Input: dimensioned drawing with shaded views. Units: mm. Origin: part minimum x, y, z. A direction names the side the tool comes from. Coordinates: 2 decimals unless noted, no trailing zeros. Write each loop counter-clockwise with the first axis right and the second up, starting at its lowest first coordinate (ties: lowest second). Pieces come first, ordered by that corner, then holes. Notation, with made-up numbers: M 60.25,10.25 L 88.25,10.25 A31 ccw 88.25,38.25 Z; hole C -33,63 d2. An arc over 180 degrees is marked long. Write each question's results on one line, items separated by ' | '. Start each with the question number.
1. First-contact query: pin 1 (4 mm diameter, centred on x = 4, y = 20.5, fed in from +Z); pin 2 (1 mm diameter, centred on x = 2, z = 33.5, fed in from +Y); pin 3 (5 mm diameter, centred on x = 4.5, y = 25, fed in from +Z). Flat tips, straight axial feed; report the tip coordinate or a pass-through.
2. Pull-direction query (Y, two-part tool) for the marked faces 1, 2 and 3; classes: +Y half, -Y half, draft (parallel to the pull), parting line (faces both ways), or undercut.
3. Section query D-D, the plane z = 30. Output: boundary loops of the cut face in (x, y), and give its area (3 significant figures).
4. Section query C-C, the plane x = 5.25. Output: boundary loops of the cut face in (y, z).
5. Section query A-A, the plane y = 20. Output: boundary loops of the cut face in (x, z).
6. Ray query, probe 1 along Y at (x, z) = (2.5, 20); probe 2 along Y at (x, z) = (6.5, 20); probe 3 along X at (y, z) = (26, 2). Return the intervals inside material, ascending.
7. Set-up query: the marked faces 4 and 5. Return all of +Z, -Z, +X, -X, +Y, -Y with unobstructed straight access to the full face (end or side cutting, diameter ignored); none if empty.
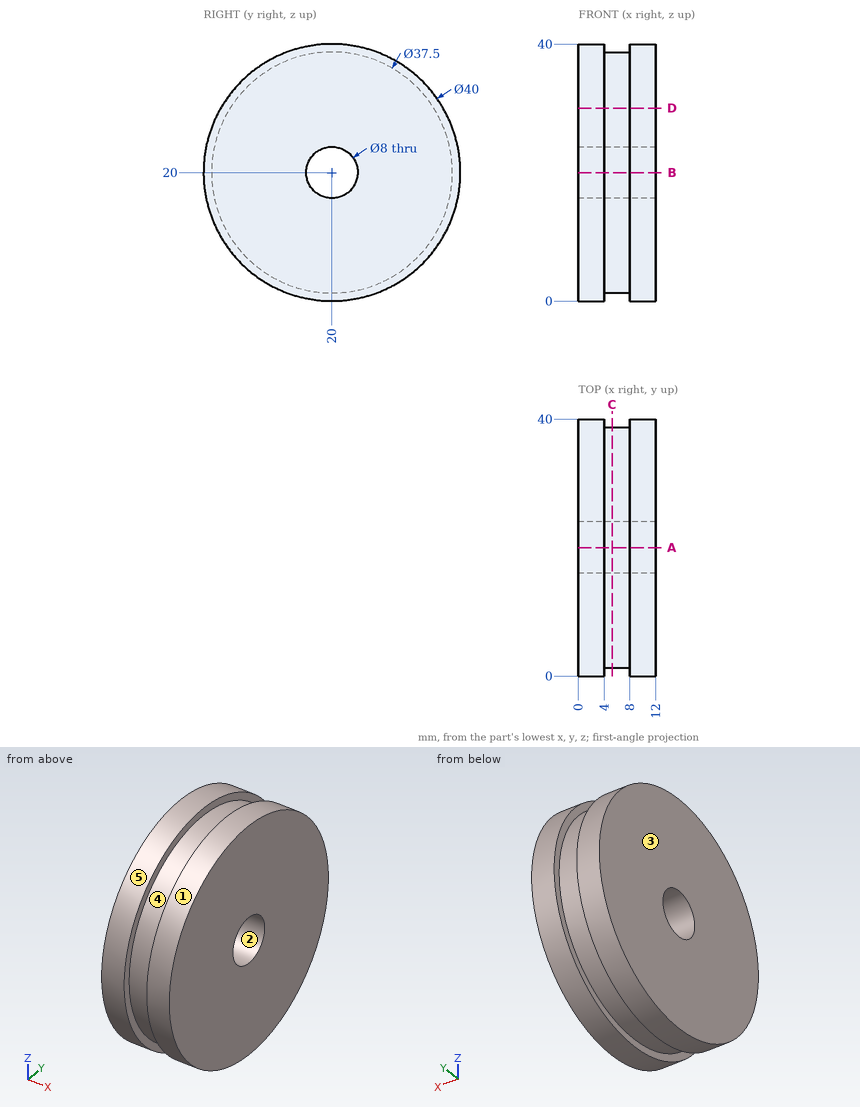
Answer:
1) pin 1: z = 40 | pin 2: y = 35.2 | pin 3: z = 39.84
2) face 1: parting line | face 2: undercut | face 3: draft
3) outline: M 0,2.68 L 4,2.68 L 4,4.14 L 8,4.14 L 8,2.68 L 12,2.68 L 12,37.32 L 8,37.32 L 8,35.86 L 4,35.86 L 4,37.32 L 0,37.32 Z | area: 404 mm^2
4) outline: C 20,20 d37.5; hole C 20,20 d8
5) outline: M 0,0 L 4,0 L 4,1.25 L 8,1.25 L 8,0 L 12,0 L 12,16 L 0,16 Z; M 0,24 L 12,24 L 12,40 L 8,40 L 8,38.75 L 4,38.75 L 4,40 L 0,40 Z
6) probe 1: 0 to 16, 24 to 40 | probe 2: 1.25 to 16, 24 to 38.75 | probe 3: 0 to 4, 8 to 12
7) face 4: none | face 5: +X, -X
